Read the model definition and answer for the solid it produces. Units are mm, in the model's axes. A direction names the side the tool comes from. Round coordinates to 2 decimals unless told otherwise and drop trailing zeros. Order: outer loops, then holes, each group sorted by start corner. A loop starts at its lowest first (then second) coordinate and runs counter-clockwise, first axis right, second up. Notation, with made-up numbers: (-1, 33.5) - (44, 33.5) arc R16 cw to (44, 51.5) - close; hole circle Ø7 at (50, 76.5). An arc over 180 degrees is marked (long way). Put each result on its own line as item: value. Start each with the question number.
Q1. Section A-A on z = 1 is taken. Give the vertices of the cut face in (x, y).
Q2. Which of the six approach directions +Z, -Z, +X, -X, +Y, -Y give full straight-line access (tool end or side, diameter ignored) to faces 1 (the face through (-243.938, 25, 89)), 2 (the face through (-254, 25, 48.612)), 3 (the face through (-42, 0, 2))?
Q3. Section C-C on y = 8 is taken. Give the vertices of the cut face in (x, z), then the cut area to 3 significant figures.
Q4. For a pull along X with two mould halves and no side action, classify faces 4 (the face through (6.062, 25, 3)), 5 (the face through (-23.938, 25, 4)), 6 (the face through (-111, 25, 148.612)), 7 (the face through (-263.938, 25, -92)) as pulls with the +X half, pulls with the -X half, needs draft (parallel to the pull), parting line crosses it, or undercut.
Q5. Section B-B on x = -227 is taken. Give the vertices of the cut face in (y, z).
Q6. Each of these flat-tipped pins is pushed along its axis until it touches: pin 1 Ø7.5 at (y, z) = (31, 18.5) entering from -X; pin 2 Ø12 at (x, z) = (-49.5, -57.5) entering from +Y. Where does it stop, or does it pass through?
Q7. Find the intervals of material crossed by line 1 along Z through (x, y) = (15.5, 20); line 2 along X through (y, z) = (45, -100.5); line 3 along Z through (x, y) = (-211.5, 3.5), in increasing order. Write a range as from..to.
from build123d import *

# Parameters (mm, degrees)
BOSS_EXTRUDE2_DEPTH = 50


with BuildPart() as part:
    # Sketch1 → Boss-Extrude2 (new body)
    with BuildSketch(Plane(origin=(0, 0, 0), x_dir=(1, 0, 0), z_dir=(0, 1, 0))):
        Polygon((46.062322946, 141.388101983), (-263.937677054, 141.388101983), (-263.937677054, 41.388101983), (-243.937677054, 41.388101983), (-243.937677054, 121.388101983), (-43.937677054, 121.388101983), (-43.937677054, -128.611898017), (-243.937677054, -128.611898017), (-243.937677054, -48.611898017), (-263.937677054, -48.611898017), (-263.937677054, -148.611898017), (46.062322946, -148.611898017), align=None)
        Polygon((26.062322946, -28.611898017), (-23.937677054, -28.611898017), (-23.937677054, 21.388101983), (26.062322946, 21.388101983), (26.062322946, 6.388101983), (6.062322946, 6.388101983), (6.062322946, -13.611898017), (26.062322946, -13.611898017), align=None, mode=Mode.SUBTRACT)
    extrude(amount=BOSS_EXTRUDE2_DEPTH)


solid = part.part
Findings:
1. outline: (-43.94, 0) - (-23.94, 0) - (-23.94, 50) - (-43.94, 50) - close; (6.06, 0) - (46.06, 0) - (46.06, 50) - (6.06, 50) - close
2. face 1: +Y, -Y
2. face 2: -X, +Y, -Y
2. face 3: +Z, -Z, +X, -X, -Y
3. outline: (-263.94, -141.39) - (46.06, -141.39) - (46.06, 148.61) - (-263.94, 148.61) - (-263.94, 48.61) - (-243.94, 48.61) - (-243.94, 128.61) - (-43.94, 128.61) - (-43.94, -121.39) - (-243.94, -121.39) - (-243.94, -41.39) - (-263.94, -41.39) - close; hole (-23.94, -21.39) - (26.06, -21.39) - (26.06, -6.39) - (6.06, -6.39) - (6.06, 13.61) - (26.06, 13.61) - (26.06, 28.61) - (-23.94, 28.61) - close
3. area: 36,000 mm2
4. face 4: undercut
4. face 5: undercut
4. face 6: needs draft
4. face 7: pulls with the -X half
5. outline: (0, -141.39) - (50, -141.39) - (50, -121.39) - (0, -121.39) - close; (0, 128.61) - (50, 128.61) - (50, 148.61) - (0, 148.61) - close
6. pin 1: x = -43.94
6. pin 2: y = 50
7. line 1: -141.39..-21.39, -6.39..13.61, 28.61..148.61
7. line 2: -263.94..-243.94, -43.94..46.06
7. line 3: -141.39..-121.39, 128.61..148.61
